Part model, mm, in its own coordinate system. A direction names the side the tool comes from. Coordinates: 2 decimals unless noted, no trailing zeros. Loops run counter-clockwise (first coordinate to the right, second up) from the corner with the lowest first, then second, coordinate; pieces in that order, holes last. Notation, with made-up numbers: (32, 43.5) - (63, 43.5) arc R4 ccw to (63, 47.5) - close; hole circle Ø7 at (63.25, 71.5). An arc over 180 degrees is marked (long way). One line per question, with ' | ' between items. Start each with the question number.
from build123d import *

# Parameters (mm, degrees)
SKETCH1_W           = 19.05
SKETCH1_H           = 19.05
SKETCH1_R           = 1.27
SKETCH1_R_2         = 3.96875
BOSS_EXTRUDE1_DEPTH = 15.875
FILLET2_R           = 3.175
SKETCH3_R           = 4.953
CUT_EXTRUDE1_DEPTH  = 9.525


with BuildPart() as part:
    # Sketch1 → Boss-Extrude1 (new body)
    with BuildSketch(Plane(origin=(0, 0, 0), x_dir=(1, 0, 0), z_dir=(0, 1, 0))):
        Rectangle(SKETCH1_W, SKETCH1_H)
        with Locations(Location((-6.35, 6.35, 0), (0, 0, 270))):
            Circle(SKETCH1_R, mode=Mode.SUBTRACT)
        with Locations(Location((6.35, 6.35, 0), (0, 0, 270))):
            Circle(SKETCH1_R, mode=Mode.SUBTRACT)
        with Locations(Location((6.35, -6.35, 0), (0, 0, 270))):
            Circle(SKETCH1_R, mode=Mode.SUBTRACT)
        with Locations(Location((-6.35, -6.35, 0), (0, 0, 270))):
            Circle(SKETCH1_R, mode=Mode.SUBTRACT)
        with Locations(Location((0, 0, 0), (0, 0, 270))):
            Circle(SKETCH1_R_2, mode=Mode.SUBTRACT)
    extrude(amount=BOSS_EXTRUDE1_DEPTH)

    # Fillet2
    fillet2_edges = [part.edges().sort_by_distance(p)[0] for p in [
        (9.525, 7.9375, 9.525),
        (-9.525, 7.9375, 9.525),
        (-9.525, 7.9375, -9.525),
        (9.525, 7.9375, -9.525),
    ]]
    fillet(fillet2_edges, radius=FILLET2_R)

    # Sketch3 → Cut-Extrude1 (cut)
    with BuildSketch(Plane(origin=(0, 15.875, 0), x_dir=(1, 0, 0), z_dir=(0, 1, 0))):
        with Locations(Location((0, 0, 0), (0, 0, 270))):
            Circle(SKETCH3_R)
    extrude(amount=-CUT_EXTRUDE1_DEPTH, mode=Mode.SUBTRACT)


solid = part.part
1) Band-saw the part on C-C on z = 0. List the corners of the cut face in (x, y) (3 decimals), then the cut area to 3 significant figures.
2) Tool access for faces 1 (the cylindrical face through (1.488, 11.179, 4.724)), 2 (the cylindrical face through (7.208, 7.826, -7.286)): list every direction of +Z, -Z, +X, -X, +Y, -Y with a clear straight run to the whole face (end or side of a thin tool).
3) Band-saw the part on D-D on z = -7. List the corners of the cut face in (x, y) (3 decimals).
4) Mould opens along X. For faces 3 (the cylindrical face through (8.57, 8.05, -8.62)), 4 (the cylindrical face through (7.61, 7.83, 6.18)), 5 (the flat face through (4, 15.875, 4)) say: +X half, -X half, draft (parallel to the pull), parting line (faces both ways), or undercut.
5) Wall check: line 1 along X through (y, z) = (11.5, -6.35) (3 decimals); line 2 along Z through (x, y) = (-6.5, 14); line 3 along Z through (x, y) = (0, 1.5) (3 decimals). Give the ranges that are in metal, low to high. Write a range as [from, to].
6) Band-saw the part on A-A on x = 0. List the corners of the cut face in (y, z) (3 decimals).
7) Band-saw the part on B-B on y = 8.5. List the corners of the cut face in (x, z) (3 decimals), then the cut area to 3 significant figures.
Values found:
1) outline: (-9.525, 0) - (-3.969, 0) - (-3.969, 6.35) - (-4.953, 6.35) - (-4.953, 15.875) - (-9.525, 15.875) - close; (3.969, 0) - (9.525, 0) - (9.525, 15.875) - (4.953, 15.875) - (4.953, 6.35) - (3.969, 6.35) - close | area: 158 mm²
2) face 1: +Y | face 2: +Y, -Y
3) outline: (-9.458, 0) - (-7.441, 0) - (-7.441, 15.875) - (-9.458, 15.875) - close; (-5.259, 0) - (5.259, 0) - (5.259, 15.875) - (-5.259, 15.875) - close; (7.441, 0) - (9.458, 0) - (9.458, 15.875) - (7.441, 15.875) - close
4) face 3: +X half | face 4: undercut | face 5: draft
5) line 1: [-9.525, -7.62], [-5.08, 5.08], [7.62, 9.525] | line 2: [-9.52, -7.61], [-5.09, 5.09], [7.61, 9.52] | line 3: [-9.525, -3.969], [3.969, 9.525]
6) outline: (0, -9.525) - (15.875, -9.525) - (15.875, -4.953) - (6.35, -4.953) - (6.35, -3.969) - (0, -3.969) - close; (0, 3.969) - (6.35, 3.969) - (6.35, 4.953) - (15.875, 4.953) - (15.875, 9.525) - (0, 9.525) - close
7) outline: (-9.525, -6.35) arc R3.175 ccw to (-6.35, -9.525) - (6.35, -9.525) arc R3.175 ccw to (9.525, -6.35) - (9.525, 6.35) arc R3.175 ccw to (6.35, 9.525) - (-6.35, 9.525) arc R3.175 ccw to (-9.525, 6.35) - close; hole circle Ø2.54 at (-6.35, -6.35); hole circle Ø2.54 at (-6.35, 6.35); hole circle Ø9.906 at (0, 0); hole circle Ø2.54 at (6.35, -6.35); hole circle Ø2.54 at (6.35, 6.35) | area: 257 mm²
